Answer from the drawing. Dimensions are ordinates in mm from the lowest x, y and z of the part. A direction names the side the tool comes from. Give positions to 0.01 mm unless a question says otherwise; leave off trailing zeros. Loops run counter-clockwise (first coordinate to the right, second up) from the corner with the lowest first, then second, coordinate; pieces in that order, holes last. Notation, with made-up numbers: (-26, 63) - (7, 63) arc R20 cw to (7, 91) - close; hole circle Ø10 at (75.25, 69.25). An arc over 180 degrees is marked (long way). One line per item, written item: value.
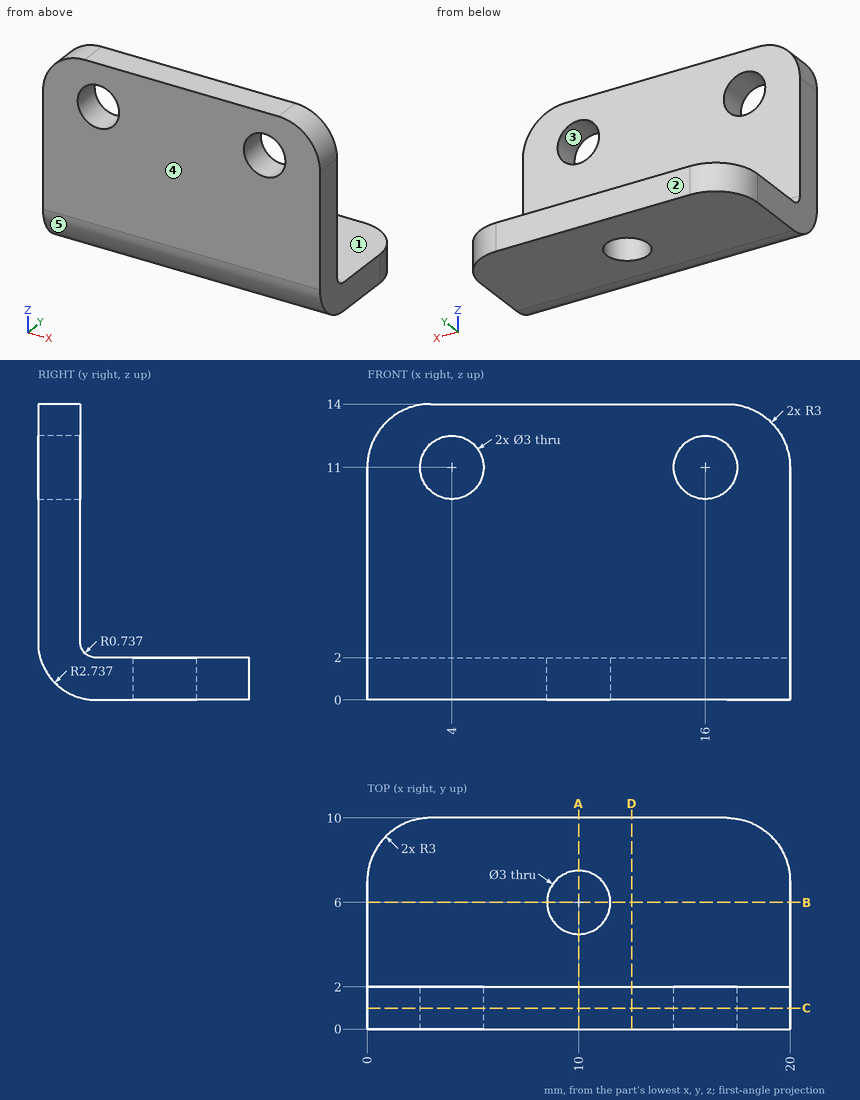
1. For the marked faces 1 and 2, determine the directions among +Z, -Z, +X, -X, +Y, -Y from which every point of the face is accessible in a straight line to the end or side of a thin tool.
Output:
face 1: +Z, +X, -X, +Y
face 2: +Z, -Z, +X, -X, +Y
2. Section A-A (x = 10) is taken. Write down the section's boundary in (y, z).
Output:
outline: (0, 2.74) arc R2.74 ccw to (2.74, 0) - (4.5, 0) - (4.5, 2) - (2.74, 2) arc R0.74 cw to (2, 2.74) - (2, 14) - (0, 14) - close; (7.5, 0) - (10, 0) - (10, 2) - (7.5, 2) - close
3. Section B-B (y = 6) is taken. Write down the section's boundary in (x, z), and give its area (3 significant figures).
Output:
outline: (0, 0) - (8.5, 0) - (8.5, 2) - (0, 2) - close; (11.5, 0) - (20, 0) - (20, 2) - (11.5, 2) - close
area: 34.0 mm²
4. The mould has two halves that part along Z. Classify the marked faces 3, 4 and 5: released by +Z, released by -Z, zero draft, split by the parting line, or undercut.
Output:
face 3: undercut
face 4: zero draft
face 5: released by -Z
5. Section C-C (y = 1) is taken. Write down the section's boundary in (x, z), and give its area (3 significant figures).
Output:
outline: (0, 0.62) - (20, 0.62) - (20, 11) arc R3 ccw to (17, 14) - (3, 14) arc R3 ccw to (0, 11) - close; hole circle Ø3 at (4, 11); hole circle Ø3 at (16, 11)
area: 250 mm²
6. Find the intervals of material crossed by line 1 along X through (y, z) = (1.05, 11); line 2 along Y through (x, z) = (15.5, 7.5), in increasing order.
Output:
line 1: x = 0 to 2.5, 5.5 to 14.5, 17.5 to 20
line 2: y = 0 to 2
7. Section D-D (x = 12.5) is taken. Write down the section's boundary in (y, z), and give its area (3 significant figures).
Output:
outline: (0, 2.74) arc R2.74 ccw to (2.74, 0) - (10, 0) - (10, 2) - (2.74, 2) arc R0.74 cw to (2, 2.74) - (2, 14) - (0, 14) - close
area: 42.5 mm²
8. Flat-ended cylindrical pins translate along their axes: pin 1 Ø5 at (x, y) = (10, 6) entering from +Z; pin 2 Ø3.5 at (x, z) = (6.5, 6.5) entering from +Y; pin 3 Ø2.5 at (x, z) = (4, 11) entering from +Y. Find the tip coordinate at first contact, or state that the pin passes through.
Output:
pin 1: stops at z = 2
pin 2: stops at y = 2
pin 3: passes through
